Geometry check sheet. Reference: the model listing, model coordinates, mm. A direction names the side the tool comes from. Round coordinates to 2 decimals unless told otherwise and drop trailing zeros. Loops run counter-clockwise (first coordinate to the right, second up) from the corner with the lowest first, then second, coordinate; pieces in that order, holes last. Notation, with made-up numbers: (-7, 2) -> (1, 2) arc R37 cw to (1, 38) -> close; hole circle Ø3 at (-9.75, 1.5). An arc over 180 degrees is marked (long way). Use a Markdown table: item, result. Add a question column.
Q1. Sectioned sample at A-A, the plane y = -9.5. Enter the section's corners in (x, z).
Q2. Sectioned sample at C-C, the plane z = 44.5. Enter the section's corners in (x, y), then the cut area to 3 significant figures.
Q3. Sectioned sample at D-D, the plane z = -18. Enter the section's corners in (x, y).
Q4. Material ranges on L1, parallel to Y at x = 5.5, z = 41; L2, parallel to Z at x = 61.5, y = -7.5; L3, parallel to X at y = -43.5, z = -34.5, recorded low to high.
Q5. Release check for a two-part mould opening along X. For faces 3 (the face through (-0.143, -37, 45.478)), 4 (the face through (6, -43, 51.917)), 5 (the face through (-18.919, -38, -30)), 6 (the face through (38.214, -63.637, 45.478)) record: released by +X, released by -X, zero draft, split by the parting line, or undercut.
Q6. Set-up check for faces 1 (the face through (70.551, -38, -3)), 2 (the face through (-51, -38, -16.357)): record each of +Z, -Z, +X, -X, +Y, -Y from which the full face is reachable in a straight line by a thin tool's end or side.
Q7. Sectioned sample at B-B, the plane x = 34.5. Enter the section's corners in (y, z).
Q8. Gauge pin test, flat ends, axial feed: P1, Ø19, axis at x = -61.5, y = -23, coming from the +Z side; P2, Ø8, axis at x = -45.5, y = -26, coming from the -Z side; P3, Ø3, axis at x = 28.5, y = -21, coming from the +Z side; P4, Ø4, axis at x = 31, z = 30.5, coming from the +Y side. Record the tip position at first contact, or that the pin passes through.
```python
from build123d import *

# Parameters (mm, degrees)
F1_DEPTH = 76.2
F2_R     = 17.175064
F2_R_2   = 8.513292
F3_DEPTH = 12.7


with BuildPart() as f1:
    # F0 (on Front) → F1 (new body)
    with BuildSketch(Plane.XZ):
        Polygon((-18.524483, 11.430001), (-81.389479, 11.430001), (-81.389479, -16.356725), (-18.918622, -16.356725), (-18.918622, -43.946382), (70.550688, -43.946382), (70.550688, 39.216723), (-18.918622, 39.216723), align=None)
    extrude(amount=F1_DEPTH)

    # F2 (on face) → F3 (join)
    with BuildSketch(Plane.XY.offset(39.216723)):
        with Locations((41.936964, -46.870772)):
            Circle(F2_R)
        with Locations((6.131807, -42.753547)):
            Circle(F2_R_2)
    extrude(amount=F3_DEPTH)


solid = f1.part
```
Values:
| question | item | result |
|---|---|---|
| 1 | outline | (-81.39, -16.36) -> (-18.92, -16.36) -> (-18.92, -43.95) -> (70.55, -43.95) -> (70.55, 39.22) -> (-18.92, 39.22) -> (-18.52, 11.43) -> (-81.39, 11.43) -> close |
| 2 | outline | circle Ø17.03 at (6.13, -42.75); circle Ø34.35 at (41.94, -46.87) |
| 2 | area | 1,150 mm^2 |
| 3 | outline | (-18.92, -76.2) -> (70.55, -76.2) -> (70.55, 0) -> (-18.92, 0) -> close |
| 4 | L1 | -51.24 to -34.26 |
| 4 | L2 | -43.95 to 39.22 |
| 4 | L3 | -18.92 to 70.55 |
| 5 | face 3 | undercut |
| 5 | face 4 | zero draft |
| 5 | face 5 | released by -X |
| 5 | face 6 | undercut |
| 6 | face 1 | +Z, -Z, +X, +Y, -Y |
| 6 | face 2 | -Z, -X, +Y, -Y |
| 7 | outline | (-76.2, -43.95) -> (0, -43.95) -> (0, 39.22) -> (-31.39, 39.22) -> (-31.39, 51.92) -> (-62.35, 51.92) -> (-62.35, 39.22) -> (-76.2, 39.22) -> close |
| 8 | P1 | z = 11.43 |
| 8 | P2 | z = -16.36 |
| 8 | P3 | z = 39.22 |
| 8 | P4 | y = 0 |
